The model under review builds one solid part; all positions refer to its coordinate system, in mm. A direction names the side the tool comes from. Coordinates: 2 decimals unless noted, no trailing zeros. Write each loop counter-clockwise with the first axis right and the second up, starting at its lowest first coordinate (ties: lowest second). Pieces come first, ordered by that corner, then holes.
1) Add section B-B, the plane x = -94.5. State the section outline as (y, z) points.
2) Machinability: for faces 1 (the flat face through (140, 39, 38)), 2 (the flat face through (-25, 43, 49)), 3 (the flat face through (156.02, 15.93, 50.7)), 4 (the flat face through (30, 17, 3)), 5 (the flat face through (30, 45, 52)), which of the approach directions +Z, -Z, +X, -X, +Y, -Y give a long, thin tool a straight path to every point of the face, cutting with its end or side? Answer none if there is none.
3) Mouldability with a two-part tool opening along Y and no side actions: class faces 6 (the flat face through (33.55, 61.44, 3.04)), 7 (the flat face through (-25, 25, 49)), 8 (the flat face through (-95.98, -20.07, 49.3)) as released by +Y, released by -Y, zero draft, split by the parting line, or undercut.
4) For line 1 (Y direction, x = 142.5, z = 52); line 2 (X direction, y = 23.5, z = 27); line 3 (Y direction, x = -8, z = 34), list the stretches that pass through material, from the lowest coordinate up.
5) Add section A-A, the plane x = 118.5. State the section outline as (y, z) points, then the cut area to 3 significant figures.
6) For P1, Ø8, axis at x = 134, y = 3.5, coming from the +Z side; P2, Ø1, axis at y = -11.5, z = 38.5, coming from the +X side; P3, Ø8, axis at x = -7.5, z = 24, coming from the -Y side, all flat-tipped, find the tip position at first contact; note any pin that passes through.
from build123d import *

# Parameters (mm, degrees)
F0_W      = 112
F0_H      = 82
F1_DEPTH  = 100
F2_T      = -3
F3_W      = 10
F3_H      = 100
F4_DEPTH  = 140
F6_DEPTH  = 100
F7_W      = 226.154828
F7_H      = 6
F8_DEPTH  = 9
F11_DEPTH = 3
F12_R     = 48.73
F13_DEPTH = 3
F14_R     = 50
F15_DEPTH = 3
F16_W     = 10
F16_H     = 100
F17_DEPTH = 140
F19_DEPTH = 82
F21_DEPTH = 3
F22_R     = 48.73
F23_DEPTH = 3
F24_R     = 50
F25_DEPTH = 3
F26_W     = 126
F26_H     = 6
F27_DEPTH = 9
F29_W     = 364
F29_H     = 6
F30_DEPTH = 9
F32_DEPTH = 372
F33_DEPTH = 356


with BuildPart() as f1:
    # F0 (on Top) → F1 (new body)
    with BuildSketch(Plane.XY):
        with Locations((31, 16)):
            Rectangle(F0_W, F0_H)
    extrude(amount=F1_DEPTH)

    # F2
    f2_openings = [f1.faces().sort_by_distance(p)[0] for p in [
        (31, 16, 100),
    ]]
    offset(amount=F2_T, openings=f2_openings)

    # F3 (on face) → F4 (join)
    with BuildSketch(Plane.YZ.offset(87)):
        with Locations((-20, 50)):
            Rectangle(F3_W, F3_H)
        with Locations((52, 50)):
            Rectangle(F3_W, F3_H)
        with Locations((34, 50)):
            Rectangle(F3_W, F3_H)
        with Locations((16, 50)):
            Rectangle(F3_W, F3_H)
        with Locations((-2, 50)):
            Rectangle(F3_W, F3_H)
    extrude(amount=F4_DEPTH)

    # F5 (on face) → F6 (cut)
    with BuildSketch(Plane.XZ.offset(25)):
        Polygon((227, 0), (227, 100), (87, 100), align=None)
    extrude(amount=-F6_DEPTH, mode=Mode.SUBTRACT)

    # F7 (on face) → F8 (join)
    with BuildSketch(Plane.XZ.offset(25)):
        with Locations((88.077414, 3)):
            Rectangle(F7_W, F7_H)
    extrude(amount=F8_DEPTH)

    # F10 (on face) → F11 (join)
    with BuildSketch(Plane.XZ.offset(-54)):
        with BuildLine():
            ThreePointArc((81, 50), (66.355339, 85.355339), (31, 100))
            Line((31, 100), (31, 0))
            ThreePointArc((31, 0), (66.355339, 14.644661), (81, 50))
        make_face()
        with BuildLine():
            Line((31, 0), (31, 100))
            ThreePointArc((31, 100), (-19, 50), (31, 0))
        make_face()
    extrude(amount=F11_DEPTH)

    # F12 (on face) → F13 (join)
    with BuildSketch(Plane.XZ.offset(-51)):
        with Locations((31, 50)):
            Circle(F12_R)
    extrude(amount=F13_DEPTH)

    # F14 (on face) → F15 (join)
    with BuildSketch(Plane.XZ.offset(-48)):
        with Locations((31, 50)):
            Circle(F14_R)
    extrude(amount=F15_DEPTH)

    # F16 (on face) → F17 (join)
    with BuildSketch(Plane(origin=(-25, 0, 0), x_dir=(0, -1, 0), z_dir=(-1, 0, 0))):
        with Locations((-52, 50)):
            Rectangle(F16_W, F16_H)
        with Locations((-34, 50)):
            Rectangle(F16_W, F16_H)
        with Locations((-16, 50)):
            Rectangle(F16_W, F16_H)
        with Locations((2, 50)):
            Rectangle(F16_W, F16_H)
        with Locations((20, 50)):
            Rectangle(F16_W, F16_H)
    extrude(amount=F17_DEPTH)

    # F18 (on face) → F19 (cut)
    with BuildSketch(Plane.XZ.offset(25)):
        Polygon((-165, 100), (-165, 0), (-25, 100), align=None)
    extrude(amount=-F19_DEPTH, mode=Mode.SUBTRACT)

    # F20 (on face) → F21 (join)
    with BuildSketch(Plane(origin=(0, -22, 0), x_dir=(-1, 0, 0), z_dir=(0, 1, 0))):
        with BuildLine():
            Line((-82.5, 50), (17.5, 50))
            ThreePointArc((17.5, 50), (-32.5, 100), (-82.5, 50))
        make_face()
        with BuildLine():
            ThreePointArc((-82.5, 50), (-32.5, 0), (17.5, 50))
            Line((17.5, 50), (-82.5, 50))
        make_face()
    extrude(amount=F21_DEPTH)

    # F22 (on face) → F23 (join)
    with BuildSketch(Plane(origin=(0, -19, 0), x_dir=(-1, 0, 0), z_dir=(0, 1, 0))):
        with Locations((-32.5, 50)):
            Circle(F22_R)
    extrude(amount=F23_DEPTH)

    # F24 (on face) → F25 (join)
    with BuildSketch(Plane(origin=(0, -16, 0), x_dir=(-1, 0, 0), z_dir=(0, 1, 0))):
        with Locations((-32.5, 50)):
            Circle(F24_R)
    extrude(amount=F25_DEPTH)

    # F26 (on face) → F27 (join)
    with BuildSketch(Plane.XZ.offset(25)):
        with Locations((-88, 3)):
            Rectangle(F26_W, F26_H)
    extrude(amount=F27_DEPTH)

    # F29 (on face) → F30 (join)
    with BuildSketch(Plane(origin=(0, 57, 0), x_dir=(-1, 0, 0), z_dir=(0, 1, 0))):
        with Locations((-31, 3)):
            Rectangle(F29_W, F29_H)
    extrude(amount=F30_DEPTH)

    # F31 (on face) → F32 (cut)
    with BuildSketch(Plane.YZ.offset(213)):
        Polygon((66, 6), (57, 6), (66, 0), align=None)
    extrude(amount=-F32_DEPTH, mode=Mode.SUBTRACT)

    # F28 (on face) → F33 (cut)
    with BuildSketch(Plane(origin=(-151, 0, 0), x_dir=(0, -1, 0), z_dir=(-1, 0, 0))):
        Polygon((34, 6), (25, 6), (34, 0), align=None)
    extrude(amount=-F33_DEPTH, mode=Mode.SUBTRACT)


solid = f1.part
Geometry results:
1. outline: (-34, 0) - (-15, 0) - (-15, 50.36) - (-25, 50.36) - (-25, 6) - close; (-7, 0) - (3, 0) - (3, 50.36) - (-7, 50.36) - close; (11, 0) - (21, 0) - (21, 50.36) - (11, 50.36) - close; (29, 0) - (39, 0) - (39, 50.36) - (29, 50.36) - close; (47, 0) - (66, 0) - (57, 6) - (57, 50.36) - (47, 50.36) - close
2. face 1: +Z, -Z, +X
2. face 2: +Z, -Z, -X
2. face 3: +Z, +X, +Y, -Y
2. face 4: none
2. face 5: +Z
3. face 6: released by +Y
3. face 7: undercut
3. face 8: zero draft
4. line 1: y = -25 to -15, -7 to 3, 11 to 21, 29 to 39, 47 to 57
4. line 2: x = -25 to -22, 84 to 87
4. line 3: y = -25 to -13, 45 to 57
5. outline: (-34, 0) - (-15, 0) - (-15, 77.5) - (-25, 77.5) - (-25, 6) - close; (-7, 0) - (3, 0) - (3, 77.5) - (-7, 77.5) - close; (11, 0) - (21, 0) - (21, 77.5) - (11, 77.5) - close; (29, 0) - (39, 0) - (39, 77.5) - (29, 77.5) - close; (47, 0) - (66, 0) - (57, 6) - (57, 77.5) - (47, 77.5) - close
5. area: 3,930 mm2
6. P1: stops at z = 69.26
6. P2: stops at x = 87
6. P3: stops at y = -25
